Build history of the part. All positions in model axes, mm. A direction names the side the tool comes from. Coordinates: 2 decimals unless noted, no trailing zeros. Loops run counter-clockwise (first coordinate to the right, second up) from the corner with the lowest first, then second, coordinate; pieces in that order, holes last. Notation, with made-up numbers: (-24, 12.5) - (8, 12.5) arc R23 cw to (8, 46.5) - close; hole circle Ø4 at (61.5, -40). An arc over 180 degrees is marked (long way). One line per item, written item: value.
```python
from build123d import *

# Parameters (mm, degrees)
SKETCH_1_W          = 70
SKETCH_1_H          = 110
EXTRUDE_1_DEPTH     = 5
EXTRUDE_2_DEPTH     = 70
SKETCH_3_W          = 12.808674266
SKETCH_3_H          = 5
CUT_EXTRUDE_1_DEPTH = 70
CUT_EXTRUDE_2_REACH = 132.806
SKETCH_4_R          = 11.2
EXTRUDE_3_DEPTH     = 20
SKETCH_6_R          = 1.5
CUT_EXTRUDE_3_DEPTH = 10
SKETCH_7_R          = 1.5
CUT_EXTRUDE_4_DEPTH = 10
CUT_EXTRUDE_5_REACH = 144.969
SKETCH_8_R          = 1.5
SKETCH_9_R          = 3
CUT_EXTRUDE_6_DEPTH = 3
CUT_EXTRUDE_7_REACH = 144.969
SKETCH_10_R         = 1
FILLET_1_R          = 4
SKETCH_11_R         = 1.5
CUT_EXTRUDE_8_DEPTH = 10


with BuildPart() as part:
    # 草图1 → 凸台-拉伸1 (new body)
    with BuildSketch(Plane(origin=(0, 0, 0), x_dir=(1, 0, 0), z_dir=(0, 1, 0))):
        with Locations((35, 55)):
            Rectangle(SKETCH_1_W, SKETCH_1_H)
    extrude(amount=EXTRUDE_1_DEPTH)

    # 草图2 → 凸台-拉伸2 (add)
    with BuildSketch(Plane(origin=(70, 0, 0), x_dir=(0, 0, -1), z_dir=(1, 0, 0))):
        with BuildLine():
            Line((12.808674266, 0), (12.808674266, -10.5))
            Line((12.808674266, -10.5), (13.225674113, -10.5))
            ThreePointArc((13.225674113, -10.5), (23.808674266, -2.500017961), (34.391674418, -10.5))
            Line((34.391674418, -10.5), (35.225674113, -10.5))
            ThreePointArc((35.225674113, -10.5), (45.808674266, -2.500017961), (56.391674418, -10.5))
            Line((56.391674418, -10.5), (57.225674113, -10.5))
            ThreePointArc((57.225674113, -10.5), (67.808674266, -2.500017961), (78.391674418, -10.5))
            Line((78.391674418, -10.5), (79.225674113, -10.5))
            ThreePointArc((79.225674113, -10.5), (83.175432131, -4.725047944), (89.808674266, -2.500017961))
            Line((89.808674266, -2.500017961), (110, -2.500017961))
            Line((110, -2.500017961), (110, 0))
            Line((110, 0), (12.808674266, 0))
        make_face()
    extrude(amount=-EXTRUDE_2_DEPTH)

    # 草图3 → 切除-拉伸1 (cut)
    with BuildSketch(Plane(origin=(70, 0, 0), x_dir=(0, 0, -1), z_dir=(1, 0, 0))):
        with Locations((6.404337133, 2.5)):
            Rectangle(SKETCH_3_W, SKETCH_3_H)
    extrude(amount=-CUT_EXTRUDE_1_DEPTH, mode=Mode.SUBTRACT)

    # 草图4 → 切除-拉伸2 (cut, up to next)
    with BuildSketch(Plane(origin=(70, 0, 0), x_dir=(0, 0, -1), z_dir=(1, 0, 0)), mode=Mode.PRIVATE) as cut_extrude_2_sk1:
        with Locations((23.808674266, -13.500017961)):
            Circle(SKETCH_4_R)
    cut_extrude_2_tool1 = extrude(cut_extrude_2_sk1.sketch, amount=-CUT_EXTRUDE_2_REACH, mode=Mode.PRIVATE) & part.part
    # 草图4 → 切除-拉伸2 (cut, up to next)
    with BuildSketch(Plane(origin=(70, 0, 0), x_dir=(0, 0, -1), z_dir=(1, 0, 0)), mode=Mode.PRIVATE) as cut_extrude_2_sk2:
        with Locations((45.808674266, -13.500017961)):
            Circle(SKETCH_4_R)
    cut_extrude_2_tool2 = extrude(cut_extrude_2_sk2.sketch, amount=-CUT_EXTRUDE_2_REACH, mode=Mode.PRIVATE) & part.part
    # 草图4 → 切除-拉伸2 (cut, up to next)
    with BuildSketch(Plane(origin=(70, 0, 0), x_dir=(0, 0, -1), z_dir=(1, 0, 0)), mode=Mode.PRIVATE) as cut_extrude_2_sk3:
        with Locations((67.808674266, -13.500017961)):
            Circle(SKETCH_4_R)
    cut_extrude_2_tool3 = extrude(cut_extrude_2_sk3.sketch, amount=-CUT_EXTRUDE_2_REACH, mode=Mode.PRIVATE) & part.part
    # 草图4 → 切除-拉伸2 (cut, up to next)
    with BuildSketch(Plane(origin=(70, 0, 0), x_dir=(0, 0, -1), z_dir=(1, 0, 0)), mode=Mode.PRIVATE) as cut_extrude_2_sk4:
        with Locations((89.808674266, -13.500017961)):
            Circle(SKETCH_4_R)
    cut_extrude_2_tool4 = extrude(cut_extrude_2_sk4.sketch, amount=-CUT_EXTRUDE_2_REACH, mode=Mode.PRIVATE) & part.part
    add(cut_extrude_2_tool1.solids().sort_by_distance((70, -13.500018, -23.808674))[0], mode=Mode.SUBTRACT)
    add(cut_extrude_2_tool2.solids().sort_by_distance((70, -13.500018, -45.808674))[0], mode=Mode.SUBTRACT)
    add(cut_extrude_2_tool3.solids().sort_by_distance((70, -13.500018, -67.808674))[0], mode=Mode.SUBTRACT)
    add(cut_extrude_2_tool4.solids().sort_by_distance((70, -13.500018, -89.808674))[0], mode=Mode.SUBTRACT)

    # 草图5 → 凸台-拉伸3 (add)
    with BuildSketch(Plane(origin=(70, 0, 0), x_dir=(0, 0, -1), z_dir=(1, 0, 0))):
        Polygon((12.808674266, 5), (110, 5), (110, -2.300017961), (110, -2.500017961), (101.008674266, -2.500017961), (101.008674266, -2.300017961), (12.808674266, -2.300017961), align=None)
    extrude(amount=EXTRUDE_3_DEPTH)

    # 草图6 → 切除-拉伸3 (cut)
    with BuildSketch(Plane.ZY):
        with Locations((-31, 0.5)):
            Circle(SKETCH_6_R)
        with Locations((-75, 0.5)):
            Circle(SKETCH_6_R)
    extrude(amount=-CUT_EXTRUDE_3_DEPTH, mode=Mode.SUBTRACT)

    # 草图7 → 切除-拉伸4 (cut)
    with BuildSketch(Plane.XY.offset(-12.808674266)):
        with Locations((12, 1.34999102)):
            Circle(SKETCH_7_R)
        with Locations((78, 1.34999102)):
            Circle(SKETCH_7_R)
    extrude(amount=-CUT_EXTRUDE_4_DEPTH, mode=Mode.SUBTRACT)

    # 草图8 → 切除-拉伸5 (cut, up to next)
    with BuildSketch(Plane(origin=(0, 5, 0), x_dir=(1, 0, 0), z_dir=(0, 1, 0)), mode=Mode.PRIVATE) as cut_extrude_5_sk1:
        with Locations(Location((78, 105.504337133, 0), (0, 0, 270))):
            Circle(SKETCH_8_R)
    cut_extrude_5_tool1 = extrude(cut_extrude_5_sk1.sketch, amount=-CUT_EXTRUDE_5_REACH, mode=Mode.PRIVATE) & part.part
    # 草图8 → 切除-拉伸5 (cut, up to next)
    with BuildSketch(Plane(origin=(0, 5, 0), x_dir=(1, 0, 0), z_dir=(0, 1, 0)), mode=Mode.PRIVATE) as cut_extrude_5_sk2:
        with Locations(Location((12, 105.504337133, 0), (0, 0, 270))):
            Circle(SKETCH_8_R)
    cut_extrude_5_tool2 = extrude(cut_extrude_5_sk2.sketch, amount=-CUT_EXTRUDE_5_REACH, mode=Mode.PRIVATE) & part.part
    add(cut_extrude_5_tool1.solids().sort_by_distance((78, 5, -105.504337))[0], mode=Mode.SUBTRACT)
    add(cut_extrude_5_tool2.solids().sort_by_distance((12, 5, -105.504337))[0], mode=Mode.SUBTRACT)

    # 草图9 → 切除-拉伸6 (cut)
    with BuildSketch(Plane(origin=(0, 5, 0), x_dir=(1, 0, 0), z_dir=(0, 1, 0))):
        with Locations(Location((78, 105.504337133, 0), (0, 0, 270))):
            Circle(SKETCH_9_R)
        with Locations(Location((12, 105.504337133, 0), (0, 0, 270))):
            Circle(SKETCH_9_R)
    extrude(amount=-CUT_EXTRUDE_6_DEPTH, mode=Mode.SUBTRACT)

    # 草图10 → 切除-拉伸7 (cut, up to next)
    with BuildSketch(Plane(origin=(0, 5, 0), x_dir=(1, 0, 0), z_dir=(0, 1, 0)), mode=Mode.PRIVATE) as cut_extrude_7_sk1:
        with Locations(Location((62.109, 103.058, 0), (0, 0, 270))):
            Circle(SKETCH_10_R)
    cut_extrude_7_tool1 = extrude(cut_extrude_7_sk1.sketch, amount=-CUT_EXTRUDE_7_REACH, mode=Mode.PRIVATE) & part.part
    add(cut_extrude_7_tool1.solids().sort_by_distance((62.109, 5, -103.058))[0], mode=Mode.SUBTRACT)

    # 圆角1
    # the kernel refuses this fillet: 4 mm, written as the material it takes off along each edge
    with BuildSketch(Plane(origin=(-10, 5, -110), x_dir=(0, -1, 0), z_dir=(1, 0, 0))) as fillet_1_piece_1:
        with BuildLine():
            CenterArc((FILLET_1_R, -FILLET_1_R), FILLET_1_R, 90, 90)
            Line((0, -FILLET_1_R), (0, 0))
            Line((0, 0), (FILLET_1_R, 0))
        make_face()
    extrude(amount=110, mode=Mode.SUBTRACT)

    # 草图11 → 切除-拉伸8 (cut)
    with BuildSketch(Plane(origin=(90, 0, 0), x_dir=(0, 0, -1), z_dir=(1, 0, 0))):
        with Locations((55, 1.34999102)):
            Circle(SKETCH_11_R)
    extrude(amount=-CUT_EXTRUDE_8_DEPTH, mode=Mode.SUBTRACT)


solid = part.part
```
Item 1: Tool access for faces 1 (the face through (76.851, 3.521, -102.733)), 2 (the face through (4.93, 0.95, -73.57)), 3 (the face through (44, -2.5, -101)): list every direction of +Z, -Z, +X, -X, +Y, -Y with a clear straight run to the whole face (end or side of a thin tool).
Check result:
face 1: +Y
face 2: -X
face 3: -Z, +X, -X, -Y
Item 2: Pull direction X, two halves, no side cores. Call faces 4 (the face through (77, 2, -107)), 5 (the face through (44, 5, -59)), 6 (the face through (70, -4, -35)): released by +X, released by -X, zero draft, split by the parting line, or undercut.
Check result:
face 4: undercut
face 5: zero draft
face 6: released by +X
Item 3: Cut at C-C, the plane x = 24. Write the cut outline in (y, z), then the cut area to 3 significant figures.
Check result:
outline: (-10.5, -79.02) arc R11.2 cw to (-2.5, -91.92) - (-2.5, -110) - (1, -110) arc R4 ccw to (5, -106) - (5, -12.81) - (-10.5, -12.81) - (-10.5, -13.02) arc R11.2 cw to (-10.5, -34.6) - (-10.5, -35.02) arc R11.2 cw to (-10.5, -56.6) - (-10.5, -57.02) arc R11.2 cw to (-10.5, -78.6) - close
area: 884 mm^2
Item 4: Probe probe 1 along Z at (x, y) = (46, -5.25); probe 2 along Y at (x, z) = (38, -93); probe 3 along Z at (x, y) = (4.5, -3.75). List the from-to ranges inside material, lowest first. Write a range as from..to.
Check result:
probe 1: z = -82.23..-75.38, -60.23..-53.38, -38.23..-31.38, -16.23..-12.81
probe 2: y = -2.5..5
probe 3: z = -84.3..-73.32, -62.3..-51.32, -40.3..-29.32, -18.3..-12.81
Item 5: Drop flat-ended pins along their axis: P1, Ø10, axis at x = 83.5, z = -71, coming from the -Y side; P2, Ø9, axis at y = -5, z = -18.5, coming from the +X side; P3, Ø1.2, axis at x = 62.109, z = -103.058, coming from the +Y side; P4, Ø0.9, axis at x = 11.5, y = 1, coming from the +Z side. Give the stop position or say it passes through.
Check result:
P1: stops at y = -2.3
P2: stops at x = 90
P3: passes through
P4: stops at z = -22.81
Item 6: Cut at A-A, the plane y = -4.75. Write the cut outline in (x, z), then the cut area to 3 significant figures.
Check result:
outline: (0, -82.82) - (70, -82.82) - (70, -74.8) - (0, -74.8) - close; (0, -60.82) - (70, -60.82) - (70, -52.8) - (0, -52.8) - close; (0, -38.82) - (70, -38.82) - (70, -30.8) - (0, -30.8) - close; (0, -16.82) - (70, -16.82) - (70, -12.81) - (0, -12.81) - close
area: 1,960 mm^2
Item 7: Cut at B-B, the plane x = 12. Write the cut outline in (y, z), then the cut area to 3 significant figures.
Check result:
outline: (-10.5, -79.02) arc R11.2 cw to (-2.5, -91.92) - (-2.5, -104) - (2, -104) - (2, -102.5) - (5, -102.5) - (5, -12.81) - (2.85, -12.81) - (2.85, -22.81) - (-0.15, -22.81) - (-0.15, -12.81) - (-10.5, -12.81) - (-10.5, -13.02) arc R11.2 cw to (-10.5, -34.6) - (-10.5, -35.02) arc R11.2 cw to (-10.5, -56.6) - (-10.5, -57.02) arc R11.2 cw to (-10.5, -78.6) - close; (-2.5, -110) - (1, -110) arc R4 ccw to (4.12, -108.5) - (2, -108.5) - (2, -107) - (-2.5, -107) - close
area: 823 mm^2
Item 8: Cut at D-D, the plane z = -55. Write the cut outline in (x, y), then the cut area to 3 significant figures.
Check result:
outline: (0, -7.1) - (70, -7.1) - (70, -2.3) - (90, -2.3) - (90, -0.15) - (80, -0.15) - (80, 2.85) - (90, 2.85) - (90, 5) - (0, 5) - close
area: 963 mm^2
